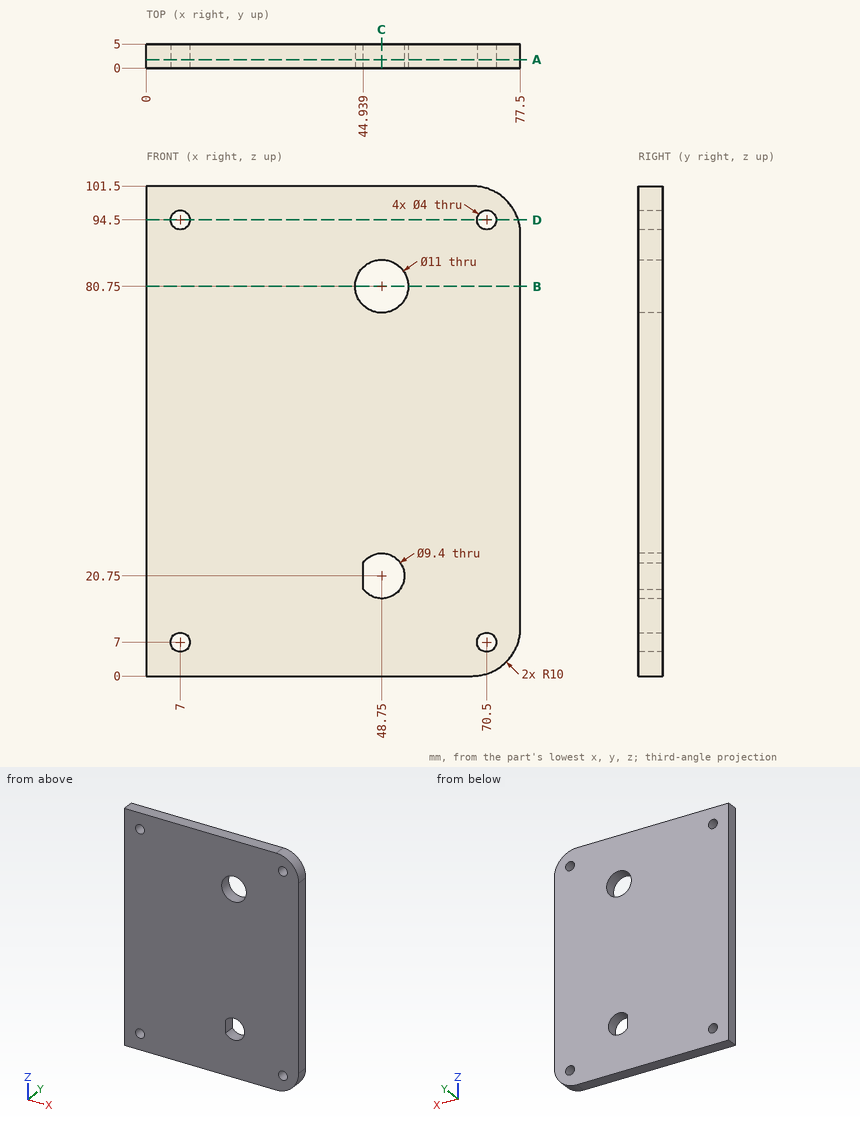
For this review, use the dimensioned drawing (mm, ordinates from the lowest corner) and the shaded views. Give positions to 0.01 mm unless a question says otherwise; leave off trailing zeros. Write each loop counter-clockwise with the first axis right and the second up, starting at its lowest first coordinate (ties: lowest second). Pieces come first, ordered by that corner, then holes. Notation, with made-up numbers: M 3.25,2.5 L 12.25,2.5 A27 cw 12.25,33.5 Z; hole C 60,51.5 d5. An arc over 180 degrees is marked long. Answer as a JSON object with one key per item and string values. Group by question number.
Item 1: For probe 1 along X at (y, z) = (2.3, 80.75); probe 2 along X at (y, z) = (2.6, 94.5); probe 3 along Z at (x, y) = (70.5, 2.55), list the stretches that pass through material, from the lowest coordinate up. Write a range as [from, to].
Item 2: Consider section D-D on z = 94.5. Write out the cut boundary in (x, y).
Item 3: Consider section A-A on y = 1.75. Write out the cut boundary in (x, z), plus the area to 3 significant figures.
Item 4: Consider section C-C on x = 48.75. Write out the cut boundary in (y, z).
Item 5: For pin 1 Ø2.5 at (x, z) = (70.5, 7) entering from -Y, flat-tipped, find the tip position at first contact; note if it passes through.
Item 6: Consider section B-B on z = 80.75. Write out the cut boundary in (x, y).
Check result:
{
 "1": {"probe 1": "x = [0, 43.25], [54.25, 77.5]", "probe 2": "x = [0, 5], [9, 68.5], [72.5, 77.04]", "probe 3": "z = [0.46, 5], [9, 92.5], [96.5, 101.04]"},
 "2": {"outline": "M 0,0 L 5,0 L 5,5 L 0,5 Z; M 9,0 L 68.5,0 L 68.5,5 L 9,5 Z; M 72.5,0 L 77.04,0 L 77.04,5 L 72.5,5 Z"},
 "3": {"outline": "M 0,0 L 67.5,0 A10 ccw 77.5,10 L 77.5,91.5 A10 ccw 67.5,101.5 L 0,101.5 Z; hole C 7,7 d4; hole C 7,94.5 d4; hole C 48.75,80.75 d11; hole M 44.94,18 A4.7 ccw long 44.94,23.5 Z; hole C 70.5,7 d4; hole C 70.5,94.5 d4", "area": "7,610 mm^2"},
 "4": {"outline": "M 0,0 L 5,0 L 5,16.05 L 0,16.05 Z; M 0,25.45 L 5,25.45 L 5,75.25 L 0,75.25 Z; M 0,86.25 L 5,86.25 L 5,101.5 L 0,101.5 Z"},
 "5": {"pin 1": "passes through"},
 "6": {"outline": "M 0,0 L 43.25,0 L 43.25,5 L 0,5 Z; M 54.25,0 L 77.5,0 L 77.5,5 L 54.25,5 Z"}
}
